Can you work these out from the drawing? Everything is in mm from the part's minimum corner. Round coordinates to 2 decimals unless told otherwise and drop trailing zeros. Loops run counter-clockwise (first coordinate to the right, second up) from the corner with the lowest first, then second, coordinate; pieces in that order, holes last. Notation, with made-up numbers: (77.5, -24) -> (117.5, -24) arc R21 cw to (117.5, -2) -> close; hole circle Ø2 at (30, 67.5). An arc over 180 degrees is marked (long way). Answer as a JSON object with one key per item and string values.
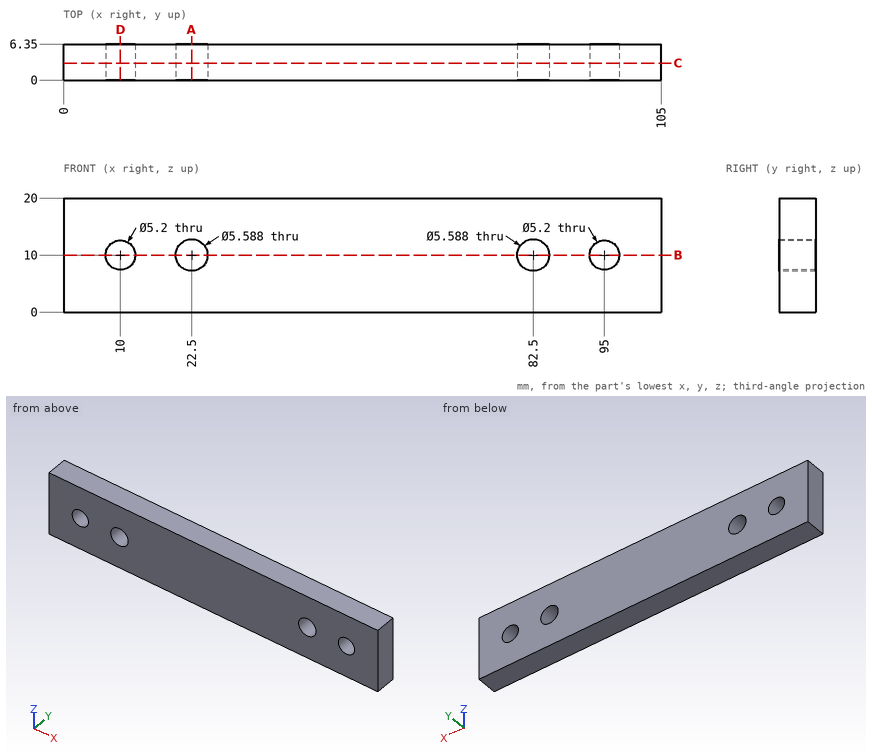
Q1. I'm going to push a flat-ended pin straight in: pin 1 (1 mm diameter, centred on x = 88, y = 5, fed in from -Z). Where does the tip first touch, or does it pass through?
Determined:
{"pin 1": "z = 0"}
Q2. I want a section at C-C, the plane y = 3. Write out the boundary of the cut face in (x, z).
Determined:
{"outline": "(0, 0) -> (105, 0) -> (105, 20) -> (0, 20) -> close; hole circle Ø5.2 at (10, 10); hole circle Ø5.59 at (22.5, 10); hole circle Ø5.59 at (82.5, 10); hole circle Ø5.2 at (95, 10)"}
Q3. I want a section at A-A, the plane x = 22.5. Write out the boundary of the cut face in (y, z).
Determined:
{"outline": "(0, 0) -> (6.35, 0) -> (6.35, 7.21) -> (0, 7.21) -> close; (0, 12.79) -> (6.35, 12.79) -> (6.35, 20) -> (0, 20) -> close"}
Q4. If I drill on L1, parallel to X at y = 2.5, z = 10; L2, parallel to Z at x = 82.5, y = 4.5; L3, parallel to Z at x = 95, y = 4, over which ranges is the centre line in solid material (lowest first)? Write a range as [from, to].
Determined:
{"L1": "[0, 7.4], [12.6, 19.71], [25.29, 79.71], [85.29, 92.4], [97.6, 105]", "L2": "[0, 7.21], [12.79, 20]", "L3": "[0, 7.4], [12.6, 20]"}
Q5. I want a section at D-D, the plane x = 10. Write out the boundary of the cut face in (y, z), then the cut area to 3 significant figures.
Determined:
{"outline": "(0, 0) -> (6.35, 0) -> (6.35, 7.4) -> (0, 7.4) -> close; (0, 12.6) -> (6.35, 12.6) -> (6.35, 20) -> (0, 20) -> close", "area": "94.0 mm²"}
Q6. I want a section at B-B, the plane z = 10. Write out the boundary of the cut face in (x, y), then the cut area to 3 significant figures.
Determined:
{"outline": "(0, 0) -> (7.4, 0) -> (7.4, 6.35) -> (0, 6.35) -> close; (12.6, 0) -> (19.71, 0) -> (19.71, 6.35) -> (12.6, 6.35) -> close; (25.29, 0) -> (79.71, 0) -> (79.71, 6.35) -> (25.29, 6.35) -> close; (85.29, 0) -> (92.4, 0) -> (92.4, 6.35) -> (85.29, 6.35) -> close; (97.6, 0) -> (105, 0) -> (105, 6.35) -> (97.6, 6.35) -> close", "area": "530 mm²"}
